Design review of the part built by this model. Coordinates are the model's own, in mm. Face numbers are marked on the shaded views. A direction names the side the tool comes from. Coordinates: 2 decimals unless noted, no trailing zeros. Loops run counter-clockwise (first coordinate to the right, second up) from the corner with the lowest first, then second, coordinate; pieces in that order, holes last. Notation, with made-up numbers: (-24.5, 59) - (31.5, 59) arc R12 ccw to (31.5, 80) - close; hole circle Ø7 at (-35, 65). An arc over 180 degrees is marked (long way). Use one line per item in the form item = value. Start each with the question number.
(1) Add section D-D (z = 2.5). State the section outline as (x, y) points (3 decimals).
(2) The part is to be moulded in two halves that separate along X. For the marked faces 4, 5 and 6, say which applies: pulls with the +X half, pulls with the -X half, needs draft (parallel to the pull), parting line crosses it, or undercut.
(3) Add section B-B (z = -6). Count the separate pieces of the cut face and the enclosed holes in it, plus the area to 3 significant figures.
(4) For L1, parallel to Y at x = -15.5, z = -7.6; L2, parallel to Z at x = 0, y = 11.5; L3, parallel to Z at x = 6, y = -6.75, list the stretches that pass through material, from the lowest coordinate up.
(5) Add section C-C (z = -12). State the section outline as (x, y) points, plus the area to 3 significant figures.
(6) Tool access review of the marked faces 1, 2 and 3: name each direction out of +Z, -Z, +X, -X, +Y, -Y from which nothing blocks a thin tool from reaching the whole face with its end or side.
(7) Add section A-A (x = -15.5). State the section outline as (y, z) points.
(8) Clearance check with flat-ended pins moving along their axes: pin 1 Ø5 at (x, y) = (-9.5, -7.5) entering from +Z; pin 2 Ø6.5 at (x, y) = (1, -9) entering from +Z; pin 3 Ø5 at (x, z) = (-2, 7) entering from +Y; pin 4 Ø5 at (x, y) = (13, -9.5) entering from -Z. State where each tip first meets the part, or that it passes through.
```python
from build123d import *

# Parameters (mm, degrees)
SKETCH_1_R          = 10
EXTRUDE_1_DEPTH     = 11.6
SKETCH_2_R          = 12.5
EXTRUDE_2_DEPTH     = 8.4
EXTRUDE_START       = -3
SKETCH_3_R          = 1.75
SKETCH_3_R_2        = 1.749999999999227
EXTRUDE_3_DEPTH     = 3
EXTRUDE_START_2     = 5.4
EXTRUDE_4_DEPTH     = 5.4
SKETCH_5_R          = 3.000000000000001
EXTRUDE_5_DEPTH     = 2
SKETCH_6_R          = 1.5000000000000002
EXTRUDE_6_DEPTH     = 8
SKETCH_7_R          = 3
EXTRUDE_7_DEPTH     = 0.8
EXTRUDE_START_3     = -11
EXTRUDE_8_DEPTH     = 11
EXTRUDE_9_DEPTH     = 8
CUT_EXTRUDE_1_DEPTH = 4.5
FILLET_1_R          = 0.5
FILLET_4_R          = 0.35
CUT_EXTRUDE_START   = -1.5
CUT_EXTRUDE_2_DEPTH = 1.5
CUT_EXTRUDE_START_2 = -0.6
SKETCH_12_R         = 10
SKETCH_12_R_2       = 9.4
CUT_EXTRUDE_3_DEPTH = 0.6
FILLET_5_R          = 0.8


with BuildPart() as part:
    # ｽｹｯﾁ1 → ﾎﾞｽ - 押し出し1 (new body)
    with BuildSketch(Plane.XY):
        Circle(SKETCH_1_R)
    extrude(amount=EXTRUDE_1_DEPTH)

    # ｽｹｯﾁ2 → ﾎﾞｽ - 押し出し2 (add)
    with BuildSketch(Plane.XY):
        Circle(SKETCH_2_R)
    extrude(amount=-EXTRUDE_2_DEPTH)

    # ｽｹｯﾁ3 → ﾎﾞｽ - 押し出し3 (add)
    # profile 1 of 4: a face of its own
    with BuildSketch(Plane(origin=(0, 0, -8.4), x_dir=(-1, 0, 0), z_dir=(0, 0, -1)).offset(EXTRUDE_START)):
        with BuildLine():
            Line((-18.500000000000004, 2.0000000000000004), (-18.500000000000004, -2.0000000000000004))
            ThreePointArc((-18.500000000000004, -2.0000000000000004), (-17.914213562373096, -3.4142135623730976), (-16.5, -4))
            Line((-16.5, -4), (-11.842719282327012, -4.000000000000001))
            ThreePointArc((-11.842719282327012, -4.000000000000001), (-12.500000000000002, 1.53e-15), (-11.842719282327012, 4.000000000000001))
            Line((-11.842719282327012, 4.000000000000001), (-16.5, 4))
            ThreePointArc((-16.5, 4), (-17.914213562373096, 3.4142135623730976), (-18.500000000000004, 2.0000000000000004))
        make_face()
        with Locations((-15.5, 0)):
            Circle(SKETCH_3_R, mode=Mode.SUBTRACT)
    # profile 2 of 4: a face of its own
    with BuildSketch(Plane(origin=(0, 0, -8.4), x_dir=(-1, 0, 0), z_dir=(0, 0, -1)).offset(EXTRUDE_START)):
        with BuildLine():
            Line((16.50000000000071, 3.999999999997067), (11.842719282327723, 3.999999999997894))
            ThreePointArc((11.842719282327723, 3.999999999997894), (12.500000000000002, -2.22183e-12), (11.842719282326302, -4.000000000002104))
            Line((11.842719282326302, -4.000000000002104), (16.49999999999929, -4.000000000002934))
            ThreePointArc((16.49999999999929, -4.000000000002934), (17.914213562372492, -3.414213562376281), (18.49999999999965, -2.000000000003289))
            Line((18.49999999999965, -2.000000000003289), (18.500000000000355, 1.999999999996712))
            ThreePointArc((18.500000000000355, 1.999999999996712), (17.9142135623737, 3.414213562369911), (16.50000000000071, 3.999999999997067))
        make_face()
        with Locations((15.5, -2.75525e-12)):
            Circle(SKETCH_3_R_2, mode=Mode.SUBTRACT)
    # profile 3 of 4: a face of its own
    with BuildSketch(Plane(origin=(0, 0, -8.4), x_dir=(-1, 0, 0), z_dir=(0, 0, -1)).offset(EXTRUDE_START)):
        with BuildLine():
            ThreePointArc((-8.311246450809406, 9.336657990625344), (-10.239400553612443, 7.1697054543880165), (-11.616202318913265, 4.616691855222107))
            ThreePointArc((-11.616202318913265, 4.616691855222107), (-13.106432708623924, 9.177222981616662), (-8.311246450809406, 9.336657990625344))
        make_face()
    # profile 4 of 4: a face of its own
    with BuildSketch(Plane(origin=(0, 0, -8.4), x_dir=(-1, 0, 0), z_dir=(0, 0, -1)).offset(EXTRUDE_START)):
        with BuildLine():
            ThreePointArc((8.311246450807749, -9.33665799062682), (10.239400553611166, -7.169705454389839), (11.616202318912443, -4.6166918552241745))
            ThreePointArc((11.616202318912443, -4.6166918552241745), (13.106432708622291, -9.177222981618991), (8.311246450807749, -9.33665799062682))
        make_face()
    extrude(amount=EXTRUDE_3_DEPTH)

    # ｽｹｯﾁ4 → ﾎﾞｽ - 押し出し4 (add)
    with BuildSketch(Plane.XY.offset(-5.400000000000001).offset(EXTRUDE_START_2)):
        with BuildLine():
            ThreePointArc((-11.616202318912443, -4.616691855224174), (-13.10643270862229, -9.17722298161899), (-8.311246450807749, -9.336657990626819))
            ThreePointArc((-8.311246450807749, -9.336657990626819), (-10.239400553611167, -7.169705454389835), (-11.616202318912443, -4.616691855224174))
        make_face()
        with BuildLine():
            ThreePointArc((11.616202318913265, 4.616691855222107), (13.106432708623922, 9.177222981616662), (8.311246450809406, 9.336657990625344))
            ThreePointArc((8.311246450809406, 9.336657990625344), (10.23940055361244, 7.169705454388018), (11.616202318913265, 4.616691855222107))
        make_face()
    extrude(amount=-EXTRUDE_4_DEPTH)

    # ｽｹｯﾁ5 → ﾎﾞｽ - 押し出し5 (add)
    with BuildSketch(Plane(origin=(0, 0, -8.4), x_dir=(-1, 0, 0), z_dir=(0, 0, -1))):
        with Locations(Location((1.1e-16, 6, 0), (0, 0, 180))):
            Circle(SKETCH_5_R)
    extrude(amount=EXTRUDE_5_DEPTH)

    # ｽｹｯﾁ6 → ﾎﾞｽ - 押し出し6 (add)
    with BuildSketch(Plane(origin=(0, 0, -10.400000000000002), x_dir=(-1, 0, 0), z_dir=(0, 0, -1))):
        with Locations((1.1e-16, 6)):
            Circle(SKETCH_6_R)
    extrude(amount=EXTRUDE_6_DEPTH)

    # ｽｹｯﾁ7 → ﾎﾞｽ - 押し出し7 (add)
    with BuildSketch(Plane.XY.offset(11.6)):
        Circle(SKETCH_7_R)
    extrude(amount=EXTRUDE_7_DEPTH)

    # ｽｹｯﾁ8 → ﾎﾞｽ - 押し出し8 (add)
    with BuildSketch(Plane.XY.offset(11.6).offset(EXTRUDE_START_3)):
        with BuildLine():
            Line((-4.215861960544603, -13.114362658155867), (7.667354864354238, -11.444285446635076))
            Line((7.667354864354238, -11.444285446635076), (7.054993220129948, -7.087105944172167))
            ThreePointArc((7.054993220129948, -7.087105944172167), (1.3917310096006568, -9.902680687415703), (-4.828223604768894, -8.757183155692958))
            Line((-4.828223604768894, -8.757183155692958), (-4.215861960544603, -13.114362658155867))
        make_face()
    extrude(amount=EXTRUDE_8_DEPTH)

    # ｽｹｯﾁ9 → ﾎﾞｽ - 押し出し9 (add)
    with BuildSketch(Plane.XY.offset(11.6)):
        Polygon((-3.4731609089884254, -13.009982832435817), (-2.9721377455321845, -16.57494787990548), (7.4256769762543025, -15.113630319824779), (6.924653812798063, -11.548665272355127), align=None)
    extrude(amount=-EXTRUDE_9_DEPTH)

    # ｽｹｯﾁ10 → ｶｯﾄ - 押し出し1 (cut)
    with BuildSketch(Plane.XY.offset(11.6)):
        Polygon((6.924653812798063, -11.548665272355127), (-3.4731609089884254, -13.009982832435817), (-2.9721377455321845, -16.57494787990548), (7.4256769762543025, -15.113630319824779), align=None)
    extrude(amount=-CUT_EXTRUDE_1_DEPTH, mode=Mode.SUBTRACT)

    # ﾌｨﾚｯﾄ1
    fillet_1_edges = [part.edges().sort_by_distance(p)[0] for p in [
        (1.7257464519048185, -12.279324052395472, 3.5999999999999996),
        (-3.4731609089884254, -13.009982832435817, 5.35),
        (6.924653812798063, -11.548665272355127, 5.35),
        (1.7257464519048185, -12.279324052395472, 7.1),
    ]]
    fillet(fillet_1_edges, radius=FILLET_1_R)

    # ﾌｨﾚｯﾄ4
    fillet_4_edges = [part.edges().sort_by_distance(p)[0] for p in [
        (11.616202318913265, 4.616691855222108, -4.200000000000001),
        (11.84271928232701, 4.000000000000002, -6.9),
        (11.84271928232701, -4.000000000000001, -6.9),
        (-11.616202318912443, -4.6166918552241745, -4.2),
        (-11.8427192823263, -4.000000000002105, -6.9),
        (-11.842719282327721, 3.999999999997894, -6.9),
    ]]
    fillet(fillet_4_edges, radius=FILLET_4_R)

    # ｽｹｯﾁ11 → ｶｯﾄ - 押し出し2 (cut)
    with BuildSketch(Plane.XY.offset(11.6).offset(CUT_EXTRUDE_START)):
        with BuildLine():
            Line((-4.828223604768897, -8.757183155692957), (-4.215861960544603, -13.114362658155867))
            Line((-4.215861960544603, -13.114362658155867), (7.667354864354238, -11.444285446635076))
            Line((7.667354864354238, -11.444285446635076), (7.054993220129944, -7.087105944172171))
            ThreePointArc((7.054993220129944, -7.087105944172171), (1.3917310096006545, -9.902680687415703), (-4.828223604768897, -8.757183155692957))
        make_face()
    extrude(amount=CUT_EXTRUDE_2_DEPTH, mode=Mode.SUBTRACT)

    # ｽｹｯﾁ12 → ｶｯﾄ - 押し出し3 (cut)
    with BuildSketch(Plane.XY.offset(11.6).offset(CUT_EXTRUDE_START_2)):
        Circle(SKETCH_12_R)
        Circle(SKETCH_12_R_2, mode=Mode.SUBTRACT)
    extrude(amount=CUT_EXTRUDE_3_DEPTH, mode=Mode.SUBTRACT)

    # ﾌｨﾚｯﾄ5
    # the kernel refuses this fillet: 0.8 mm, written as the material it takes off along each edge
    with BuildSketch(Plane(origin=(0, 0, 11), x_dir=(0.7054993220130121, -0.7087105944171995, 0), z_dir=(-0.7087105944171995, -0.7054993220130121, 0))) as fillet_5_piece_1:
        with BuildLine():
            CenterArc((9.200000000000001, -0.7745966692414843), FILLET_5_R, 0, 75.52248781407015)
            Line((9.4, 0), (9.404000000000002, 0.01549193338482979))
            ThreePointArc((9.404000000000002, 0.01549193338482979), (9.700000000000001, 0.01600000000000001), (10, 0.01600000000000001))
            Line((10, 0.01600000000000001), (10.016, 0))
            Line((10.016, 0), (10.016, -0.7745966692414843))
            Line((10.016, -0.7745966692414843), (10, -0.7745966692414843))
        make_face()
    revolve(axis=Axis((0, 0, 11), (0, 0, 1)), revolution_arc=45.130102354154545, mode=Mode.SUBTRACT)
    with BuildSketch(Plane(origin=(0, 0, 11), x_dir=(-0.48282236047689747, -0.8757183155692913, 0), z_dir=(-0.8757183155692913, 0.48282236047689747, 0))) as fillet_5_piece_2:
        with BuildLine():
            CenterArc((9.200000000000001, -0.7745966692414824), FILLET_5_R, 0, 75.52248781407025)
            Line((10.000000000000002, -0.7745966692414824), (10.016000000000002, -0.7745966692414824))
            Line((10.016000000000002, -0.7745966692414824), (10.016, 0))
            Line((10.016, 0), (10, 0.01600000000000001))
            ThreePointArc((10, 0.01600000000000001), (9.699999999999998, 0.01600000000000001), (9.404, 0.01549193338483157))
            Line((9.404, 0.01549193338483157), (9.399999999999999, 1.78e-15))
        make_face()
    revolve(axis=Axis((0, 0, 11), (0, 0, 1)), revolution_arc=73.73979529168996, mode=Mode.SUBTRACT)
    with BuildSketch(Plane(origin=(0, 0, 11), x_dir=(1, 0, 0), z_dir=(0, -1, 0))) as fillet_5_piece_3:
        with BuildLine():
            CenterArc((9.2, -0.7745966692414825), FILLET_5_R, 0, 75.52248781406999)
            Line((9.4, 0), (9.404, 0.01549193338482979))
            ThreePointArc((9.404, 0.01549193338482979), (9.7, 0.01600000000000001), (10, 0.01600000000000001))
            Line((10, 0.01600000000000001), (10.016, 0))
            Line((10.016, 0), (10.016, -0.7745966692414825))
            Line((10.016, -0.7745966692414825), (10, -0.7745966692414825))
        make_face()
    revolve(axis=Axis((0, 0, 11), (0, 0, 1)), revolution_arc=241.1301023541555, mode=Mode.SUBTRACT)


solid = part.part
```
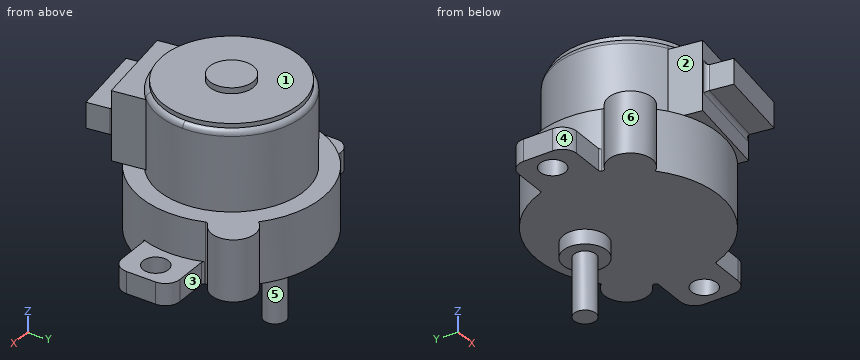
Computed values:
q1.outline = (-4.828, -8.757) - (-4.216, -13.114) - (7.667, -11.444) - (7.055, -7.087) arc R10 ccw (long way) to start
q2.face_4 = pulls with the -X half
q2.face_5 = parting line crosses it
q2.face_6 = undercut
q3.separate_pieces = 1
q3.enclosed_holes = 2
q3.area = 603 mm^2
q4.L1 = -4 to -1.75, 1.75 to 4
q4.L2 = -8.4 to 0
q4.L3 = -8.4 to 11.6
q5.outline = circle Ø3 at (0, 6)
q5.area = 7.07 mm^2
q6.face_1 = +Z
q6.face_2 = +Z, -X, -Y
q6.face_3 = +Z, -Z, +X
q7.outline = (-4, -8.4) - (-1.75, -8.4) - (-1.75, -5.4) - (-4, -5.4) - close; (1.75, -8.4) - (4, -8.4) - (4, -5.4) - (1.75, -5.4) - close
q8.pin_1 = 10.92
q8.pin_2 = 11.6
q8.pin_3 = 10
q8.pin_4 = through
